Can you work these out from the model? Positions are in its coordinate system, mm. Face numbers are marked on the shaded views. A direction names the side the tool comes from. Round coordinates to 2 decimals unless told otherwise and drop trailing zeros. Loops run counter-clockwise (first coordinate to the right, second up) from the corner with the lowest first, then second, coordinate; pieces in that order, holes last.
(1) I want a section at C-C on x = -69. Write out the boundary of the cut face in (y, z).
(2) I want a section at A-A on y = 0. Write out the boundary of the cut face in (x, z), plus the area to 3 significant figures.
(3) I want a section at B-B on z = 6. Write out the boundary of the cut face in (x, y).
(4) Will these pins go through, and if not, where does the flat tip stop? pin 1 Ø1.5 at (x, y) = (-4.5, -3) entering from -Z; pin 2 Ø20 at (x, y) = (-20, 1.5) entering from +Z.
(5) If I drill on line 1 along Y through (x, z) = (-97, 10); line 2 along Z through (x, y) = (-3, -9.5); line 3 along X through (y, z) = (5.5, 6), over which ranges is the centre line in solid material (lowest first)?
(6) Which directions (+Z, -Z, +X, -X, +Y, -Y) give clear straight access to the entire face, cutting with the end or side of a thin tool? Please do the marked faces 1 and 2.
(7) I want a section at D-D on y = 13. Write out the boundary of the cut face in (x, z), plus the area to 3 significant figures.
(8) Thinking about a two-plate mould opening in Y: for the marked faces 3, 4 and 5, which applies, released by +Y, released by -Y, zero draft, split by the parting line, or undercut?
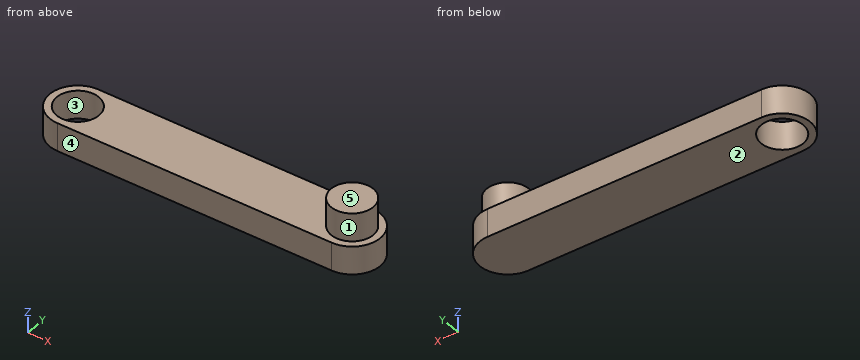
from build123d import *

# Parameters (mm, degrees)
BOSS_EXTRUDE1_DEPTH = 20
SKETCH2_R           = 15
CUT_EXTRUDE1_DEPTH  = 20
SKETCH3_R           = 15
BOSS_EXTRUDE2_DEPTH = 20


with BuildPart() as part:
    # Sketch1 → Boss-Extrude1 (new body)
    with BuildSketch(Plane.XY):
        with BuildLine():
            Line((97.5, 20), (-97.5, 20))
            ThreePointArc((-97.5, 20), (-117.5, 0), (-97.5, -20))
            Line((-97.5, -20), (97.5, -20))
            ThreePointArc((97.5, -20), (117.5, 0), (97.5, 20))
        make_face()
    extrude(amount=BOSS_EXTRUDE1_DEPTH)

    # Sketch2 → Cut-Extrude1 (cut)
    with BuildSketch(Plane.XY.offset(20)):
        with Locations((-97.5, 0)):
            Circle(SKETCH2_R)
    extrude(amount=-CUT_EXTRUDE1_DEPTH, mode=Mode.SUBTRACT)

    # Sketch3 → Boss-Extrude2 (add)
    with BuildSketch(Plane.XY.offset(20)):
        with Locations((97.5, 0)):
            Circle(SKETCH3_R)
    extrude(amount=BOSS_EXTRUDE2_DEPTH)


solid = part.part
Filled sheet:
1. outline: (-20, 0) - (20, 0) - (20, 20) - (-20, 20) - close
2. outline: (-117.5, 0) - (-112.5, 0) - (-112.5, 20) - (-117.5, 20) - close; (-82.5, 0) - (117.5, 0) - (117.5, 20) - (112.5, 20) - (112.5, 40) - (82.5, 40) - (82.5, 20) - (-82.5, 20) - close
2. area: 4,700 mm2
3. outline: (-97.5, -20) - (97.5, -20) arc R20 ccw to (97.5, 20) - (-97.5, 20) arc R20 ccw to start; hole circle Ø30 at (-97.5, 0)
4. pin 1: stops at z = 0
4. pin 2: stops at z = 20
5. line 1: y = -20 to -14.99, 14.99 to 20
5. line 2: z = 0 to 20
5. line 3: x = -116.73 to -111.46, -83.54 to 116.73
6. face 1: +Z
6. face 2: -Z, +X, -X, +Y, -Y
7. outline: (-112.7, 0) - (-104.98, 0) - (-104.98, 20) - (-112.7, 20) - close; (-90.02, 0) - (112.7, 0) - (112.7, 20) - (104.98, 20) - (104.98, 40) - (90.02, 40) - (90.02, 20) - (-90.02, 20) - close
7. area: 4,510 mm2
8. face 3: undercut
8. face 4: released by -Y
8. face 5: zero draft
